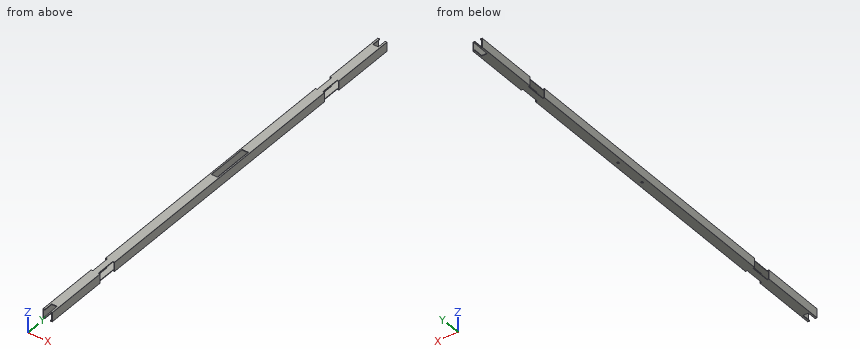
```python
from build123d import *

# Parameters (mm, degrees)
SKETCH1_W           = 17
SKETCH1_H           = 17
BOSS_EXTRUDE1_DEPTH = 977
SKETCH2_W           = 12
SKETCH2_H           = 20
CUT_EXTRUDE1_DEPTH  = 1177
SKETCH3_W           = 4
SKETCH3_H           = 42.2
CUT_EXTRUDE2_DEPTH  = 1177
SKETCH7_W           = 14
SKETCH7_H           = 90
CUT_EXTRUDE5_DEPTH  = 10
SKETCH8_R           = 2.5
CUT_EXTRUDE6_DEPTH  = 10


with BuildPart() as part:
    # Sketch1 → Boss-Extrude1 (new body)
    with BuildSketch(Plane(origin=(0, 0, 0), x_dir=(1, 0, 0), z_dir=(0, 1, 0))):
        with BuildLine():
            Line((0.5, 0), (19.5, 0))
            ThreePointArc((19.5, 0), (19.853553391, 0.146446609), (20, 0.5))
            Line((20, 0.5), (20, 19.5))
            ThreePointArc((20, 19.5), (19.853553391, 19.853553391), (19.5, 20))
            Line((19.5, 20), (0.5, 20))
            ThreePointArc((0.5, 20), (0.146446609, 19.853553391), (0, 19.5))
            Line((0, 19.5), (0, 0.5))
            ThreePointArc((0, 0.5), (0.146446609, 0.146446609), (0.5, 0))
        make_face()
        with Locations((10, 10)):
            Rectangle(SKETCH1_W, SKETCH1_H, mode=Mode.SUBTRACT)
    extrude(amount=BOSS_EXTRUDE1_DEPTH)

    # Sketch2 → Cut-Extrude1 (cut)
    with BuildSketch(Plane.XY):
        with Locations((10, 967)):
            Rectangle(SKETCH2_W, SKETCH2_H)
    cut_extrude1 = extrude(amount=-CUT_EXTRUDE1_DEPTH, mode=Mode.SUBTRACT)

    # Sketch3 → Cut-Extrude2 (cut)
    with BuildSketch(Plane(origin=(0, 0, -20), x_dir=(-1, 0, 0), z_dir=(0, 0, -1))):
        with Locations((-2, 815.9)):
            Rectangle(SKETCH3_W, SKETCH3_H)
        with Locations((-18, 815.9)):
            Rectangle(SKETCH3_W, SKETCH3_H)
    cut_extrude2 = extrude(amount=-CUT_EXTRUDE2_DEPTH, mode=Mode.SUBTRACT)

    # Mirror1: Cut-Extrude1, Cut-Extrude2 across plane
    add(cut_extrude1.mirror(Plane.ZX.offset(488.5)), mode=Mode.SUBTRACT)
    add(cut_extrude2.mirror(Plane.ZX.offset(488.5)), mode=Mode.SUBTRACT)

    # Sketch7 → Cut-Extrude5 (cut)
    with BuildSketch(Plane.XY):
        with Locations((10, 532)):
            Rectangle(SKETCH7_W, SKETCH7_H)
    extrude(amount=-CUT_EXTRUDE5_DEPTH, mode=Mode.SUBTRACT)

    # Sketch8 → Cut-Extrude6 (cut)
    with BuildSketch(Plane.XY.offset(-18.5)):
        with Locations((10, 567)):
            Circle(SKETCH8_R)
        with Locations((10, 497)):
            Circle(SKETCH8_R)
    extrude(amount=-CUT_EXTRUDE6_DEPTH, mode=Mode.SUBTRACT)


solid = part.part
```
The model under review builds one solid part; all positions refer to its coordinate system, in mm. Round coordinates to 2 decimals unless told otherwise and drop trailing zeros. Order: outer loops, then holes, each group sorted by start corner. A loop starts at its lowest first (then second) coordinate and runs counter-clockwise, first axis right, second up. Notation, with made-up numbers: M 36.5,55.5 L 78.5,55.5 A25 cw 78.5,88.5 Z; hole C 73,39.5 d10. An arc over 180 degrees is marked long. Use a Markdown table: item, result.
1) Wall thickness on line 1 along Y through (x, z) = (10, -19); line 2 along Z through (x, y) = (3.25, 363); line 3 along X through (y, z) = (567, -19.25): over which ranges is each line inside the solid? List them lowest first. Write a range as [from, to].
Report:
| item | result |
|---|---|
| line 1 | [20, 494.5], [499.5, 564.5], [569.5, 957] |
| line 2 | [-20, -18.5], [-1.5, 0] |
| line 3 | [0, 7.5], [12.5, 20] |
2) Insertion check: pin 1 (4 mm diameter, centred on x = 15.5, z = -9, fed in from +Y); pin 2 (1.6 mm diameter, centred on x = 12, z = -0.5, fed in from -Y). Each pin has a flat end and moves straight along its axis. Give the tip position at first contact, or say it passes through.
Report:
| item | result |
|---|---|
| pin 1 | through |
| pin 2 | y = 20 |
3) Consider section B-B (y = 467). Write out the cut boundary in (x, z).
Report:
| item | result |
|---|---|
| outline | M 0,-19.5 A0.5 ccw 0.5,-20 L 19.5,-20 A0.5 ccw 20,-19.5 L 20,-0.5 A0.5 ccw 19.5,0 L 0.5,0 A0.5 ccw 0,-0.5 Z; hole M 1.5,-18.5 L 18.5,-18.5 L 18.5,-1.5 L 1.5,-1.5 Z |
4) Consider section A-A (z = -9). Write out the cut boundary in (x, y), then the cut area to 3 significant figures.
Report:
| item | result |
|---|---|
| outline | M 0,0 L 1.5,0 L 1.5,140 L 0,140 Z; M 0,182.2 L 1.5,182.2 L 1.5,794.8 L 0,794.8 Z; M 0,837 L 1.5,837 L 1.5,977 L 0,977 Z; M 18.5,0 L 20,0 L 20,140 L 18.5,140 Z; M 18.5,182.2 L 20,182.2 L 20,794.8 L 18.5,794.8 Z; M 18.5,837 L 20,837 L 20,977 L 18.5,977 Z |
| area | 2,680 mm^2 |
